The listing builds one solid part. Answer for the finished solid, in the listing's coordinates (mm). A direction names the side the tool comes from. Coordinates: 2 decimals unless noted, no trailing zeros. Order: outer loops, then holes, each group sorted by start corner. A loop starts at its lowest first (then second) coordinate and runs counter-clockwise, first axis right, second up. Notation, with made-up numbers: (86.25, -12) -> (122.25, -12) arc R8 cw to (122.25, 2) -> close; hole circle Ø7 at (-36, 67). An arc over 180 degrees is marked (long way). Write item = value, one per line. Start each with the question number.
```python
from build123d import *

# Parameters (mm, degrees)
BOSS_EXTRUDE1_DEPTH     = 2.125
BOSS_EXTRUDE3_START     = -0.4
BOSS_EXTRUDE3_OUTLINE_W = 36
BOSS_EXTRUDE3_OUTLINE_H = 16.5
BOSS_EXTRUDE3_DEPTH     = 0.4
FILLET1_R               = 4
FILLET2_R               = 4
FILLET3_R               = 0.3
FILLET4_R               = 0.4


# Read off the part's stored shape, not the designer's step: Boss-Extrude3
with BuildPart() as part:
    # Sketch1 → Boss-Extrude1 (new body)
    with BuildSketch(Plane(origin=(0, 0, 0), x_dir=(1, 0, 0), z_dir=(0, 1, 0))):
        with BuildLine():
            Line((-9.970479705, 7.970479705), (7.029520295, 7.970479705))
            ThreePointArc((7.029520295, 7.970479705), (13.529520295, 1.470479705), (7.029520295, -5.029520295))
            Line((7.029520295, -5.029520295), (-9.970479705, -5.029520295))
            ThreePointArc((-9.970479705, -5.029520295), (-16.470479705, 1.470479705), (-9.970479705, 7.970479705))
        make_face()
        with BuildLine():
            Line((-9.970479705, 6.970479705), (7.029520295, 6.970479705))
            ThreePointArc((7.029520295, 6.970479705), (12.529520295, 1.470479705), (7.029520295, -4.029520295))
            Line((7.029520295, -4.029520295), (-9.970479705, -4.029520295))
            ThreePointArc((-9.970479705, -4.029520295), (-15.470479705, 1.470479705), (-9.970479705, 6.970479705))
        make_face(mode=Mode.SUBTRACT)
    extrude(amount=BOSS_EXTRUDE1_DEPTH)

    # Boss-Extrude3 outline → Boss-Extrude3 (add)
    with BuildSketch(Plane(origin=(0, 0, 0), x_dir=(1, 0, 0), z_dir=(0, 1, 0)).offset(BOSS_EXTRUDE3_START)):
        with Locations((-1.470479705, 1.470479705)):
            Rectangle(BOSS_EXTRUDE3_OUTLINE_W, BOSS_EXTRUDE3_OUTLINE_H)
        with BuildLine():
            Line((7.029520295, -4.029520295), (-9.970479705, -4.029520295))
            ThreePointArc((-9.970479705, -4.029520295), (-15.470479705, 1.470479705), (-9.970479705, 6.970479705))
            Line((-9.970479705, 6.970479705), (7.029520295, 6.970479705))
            ThreePointArc((7.029520295, 6.970479705), (12.529520295, 1.470479705), (7.029520295, -4.029520295))
        make_face(mode=Mode.SUBTRACT)
    extrude(amount=BOSS_EXTRUDE3_DEPTH)

    # Fillet1
    fillet1_edges = [part.edges().sort_by_distance(p)[0] for p in [
        (-19.470479705, -0.2, 6.779520295),
    ]]
    fillet(fillet1_edges, radius=FILLET1_R)

    # Fillet2
    fillet2_edges = [part.edges().sort_by_distance(p)[0] for p in [
        (16.529520295, -0.2, 6.779520295),
        (-19.470479705, -0.2, -9.720479705),
        (16.529520295, -0.2, -9.720479705),
    ]]
    fillet(fillet2_edges, radius=FILLET2_R)

    # Fillet3
    fillet3_edges = [part.edges().sort_by_distance(p)[0] for p in [
        (13.529520295, 2.125, -1.470479705),
        (-1.470479705, 2.125, -7.970479705),
        (-16.470479705, 2.125, -1.470479705),
        (-1.470479705, 2.125, 5.029520295),
    ]]
    fillet(fillet3_edges, radius=FILLET3_R)

    # Fillet4
    fillet4_edges = [part.edges().sort_by_distance(p)[0] for p in [
        (-1.470479705, 0, -7.970479705),
        (13.529520295, 0, -1.470479705),
        (-1.470479705, 0, 5.029520295),
        (-16.470479705, 0, -1.470479705),
    ]]
    fillet(fillet4_edges, radius=FILLET4_R)


solid = part.part
```
Item 1: Section A-A, the plane x = 3 is taken. Give the vertices of the cut face in (y, z) (3 decimals).
Item 2: Consider probe 1 along Z at (x, y) = (-5.5, 0.35); probe 2 along Z at (x, y) = (3, -0.1); probe 3 along Y at (x, z) = (8, 6). Determine where each line is inside the solid, lowest interval first.
Item 3: Which of the six approach directions +Z, -Z, +X, -X, +Y, -Y give full straight-line access (tool end or side, diameter ignored) to faces 1 (the cylindrical face through (13.53, 1.1, -1.61)), 2 (the flat face through (-2, 1, -7.97)), 3 (the flat face through (-1, 1, 4.03)), 4 (the flat face through (-1, 1, 5.03)), 5 (the flat face through (-2, 0, 6))?
Item 4: Section B-B, the plane y = 0.75 is taken. Give the vertices of the cut face in (x, z).
Item 5: For a pull along Z with two mould halves and no side action, classify faces 6 (the cylindrical face through (-18.33, -0.2, -8.52)), 7 (the cylindrical face through (-15.47, 0.84, -1.35)), 8 (the cylindrical face through (-16.47, 1.1, -1.33)) as pulls with the +Z half, pulls with the -Z half, needs draft (parallel to the pull), parting line crosses it, or undercut.
Item 6: This flat-tipped pin is pushed along its axis until it touches: pin 1 (1 mm diameter, centred on x = -7, y = 1, fed in from +Z). Where does it stop, or does it pass through?
A:
q1.outline = (-0.4, -9.72) -> (0, -9.72) -> (0, -8.37) arc R0.4 cw to (0.4, -7.97) -> (1.825, -7.97) arc R0.3 ccw to (2.125, -7.67) -> (2.125, -6.97) -> (-0.4, -6.97) -> close; (-0.4, 4.03) -> (2.125, 4.03) -> (2.125, 4.73) arc R0.3 ccw to (1.825, 5.03) -> (0.4, 5.03) arc R0.4 cw to (0, 5.43) -> (0, 6.78) -> (-0.4, 6.78) -> close
q2.probe_1 = -7.97 to -6.97, 4.03 to 5.03
q2.probe_2 = -9.72 to -6.97, 4.03 to 6.78
q2.probe_3 = -0.4 to 0
q3.face_1 = +X, +Y
q3.face_2 = -Z, +X, -X, +Y
q3.face_3 = +Y, -Y
q3.face_4 = +Z, +X, -X, +Y
q3.face_5 = +Y
q4.outline = (-9.97, -7.97) -> (7.03, -7.97) arc R6.5 ccw to (7.03, 5.03) -> (-9.97, 5.03) arc R6.5 ccw to start; hole (-9.97, -6.97) -> (7.03, -6.97) arc R5.5 ccw to (7.03, 4.03) -> (-9.97, 4.03) arc R5.5 ccw to start
q5.face_6 = pulls with the -Z half
q5.face_7 = undercut
q5.face_8 = parting line crosses it
q6.pin_1 = 5.03
